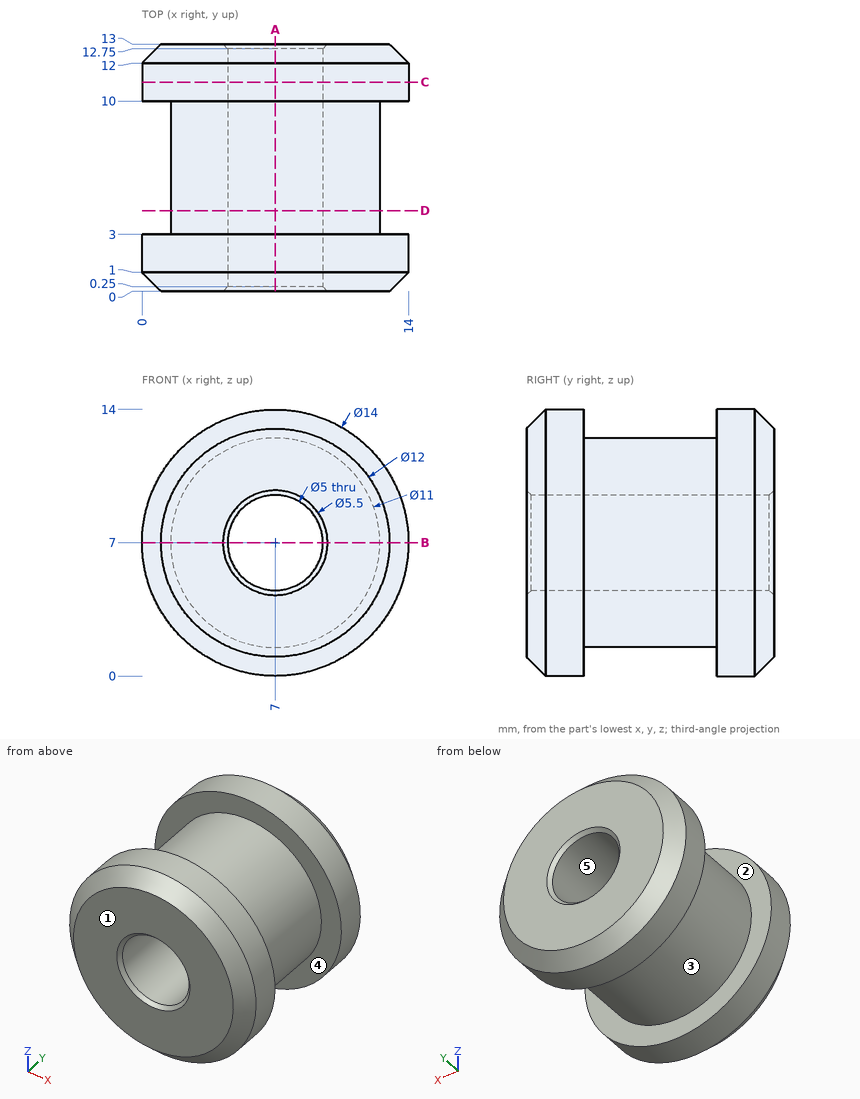
Job drawing, mm, ordinate dimensions from the low corner. One solid piece. A direction names the side the tool comes from. Give positions to 0.01 mm unless a question says otherwise; leave off trailing zeros. Order: outer loops, then holes, each group sorted by start corner. A loop starts at its lowest first (then second) coordinate and runs counter-clockwise, first axis right, second up. Notation, with made-up numbers: (-36.5, 42.5) - (-19.5, 42.5) arc R21 ccw to (-19.5, 51.5) - close; hole circle Ø2 at (-14.75, 62.25). An arc over 180 degrees is marked (long way). Return JSON: item names as keys, results as strings.
1) Pull direction X, two halves, no side cores. Call the marked faces 3, 4 and 5: pulls with the +X half, pulls with the -X half, needs draft (parallel to the pull), parting line crosses it, or undercut.
Geometry says:
{"face 3": "parting line crosses it", "face 4": "needs draft", "face 5": "undercut"}
2) 3-axis set-ups, long thin cutter, end or side, ignore diameter. For the marked faces 1 and 2: which of +Z, -Z, +X, -X, +Y, -Y reach the whole face in a straight line?
Geometry says:
{"face 1": "+Z, -Z, +X, -X, -Y", "face 2": "none"}
3) Probe line 1 (Y direction, x = 10.5, z = 11.75); line 2 (X direction, y = 4, z = 7); line 3 (Y direction, x = 2.25, z = 10.75). List the from-to ranges inside material, lowest first. Write a range as from..to.
Geometry says:
{"line 1": "0..3, 10..13", "line 2": "1.5..4.5, 9.5..12.5", "line 3": "0.05..3, 10..12.95"}
4) Cut at B-B, the plane z = 7. Give the cut face in (x, y).
Geometry says:
{"outline": "(0, 1) - (1, 0) - (4.25, 0) - (4.5, 0.25) - (4.5, 12.75) - (4.25, 13) - (1, 13) - (0, 12) - (0, 10) - (1.5, 10) - (1.5, 3) - (0, 3) - close; (9.5, 0.25) - (9.75, 0) - (13, 0) - (14, 1) - (14, 3) - (12.5, 3) - (12.5, 10) - (14, 10) - (14, 12) - (13, 13) - (9.75, 13) - (9.5, 12.75) - close"}
5) Cut at C-C, the plane y = 11. Give the cut face in (x, z), plus the area to 3 significant figures.
Geometry says:
{"outline": "circle Ø14 at (7, 7); hole circle Ø5 at (7, 7)", "area": "134 mm²"}
6) Flat gauge pins, fed straight in: P1, Ø2, axis at x = 2.5, y = 3, coming from the +Z side; P2, Ø1, axis at y = 6, z = 3, coming from the -X side. Where does each tip first touch, or does it go through?
Geometry says:
{"P1": "z = 13.06", "P2": "x = 2.76"}
7) Cut at A-A, the plane x = 7. Give the cut face in (y, z), plus the area to 3 significant figures.
Geometry says:
{"outline": "(0, 1) - (1, 0) - (3, 0) - (3, 1.5) - (10, 1.5) - (10, 0) - (12, 0) - (13, 1) - (13, 4.25) - (12.75, 4.5) - (0.25, 4.5) - (0, 4.25) - close; (0, 9.75) - (0.25, 9.5) - (12.75, 9.5) - (13, 9.75) - (13, 13) - (12, 14) - (10, 14) - (10, 12.5) - (3, 12.5) - (3, 14) - (1, 14) - (0, 13) - close", "area": "93.9 mm²"}
8) Cut at D-D, the plane y = 4.25. Give the cut face in (x, z), plus the area to 3 significant figures.
Geometry says:
{"outline": "circle Ø11 at (7, 7); hole circle Ø5 at (7, 7)", "area": "75.4 mm²"}
